Autodesk Inventor part; units mm, degrees
ref_plane "dia1_XY" through (0, 3.175, 0) normal (1, 0, 0) x (0, 0, -1)
ref_plane "dia1_YZ" through (0, 3.175, 0) normal (0, 0, -1) x (0, 1, 0)
ref_plane "dia1_ZX" through (0, 3.175, 0) normal (0, 1, 0) x (1, 0, 0)
sketch "Sketch_1" plane through (0, 0, 0) normal (0, 0, 1) x (1, 0, 0)
  line L0 (87.3252, 0) -> (0, 0)
  line L1 (0, 0) -> (0, 3.175)
  line L2 (0, 3.175) -> (65.8876, 3.175)
  line L3 (65.8876, 3.175) -> (65.8876, 9.6202)
  line L4 (65.8876, 9.6202) -> (87.3252, 9.6202)
  line L5 (87.3252, 9.6202) -> (87.3252, 0)
  line L6 (87.3252, 0) -> (0, 0)
revolve "Revolution1" add sketch "Sketch_1" angle 360 about axis through (87.3252, 0, 0) along (1, 0, 0)
sketch "Sketch_3" plane through (0, 0, 0) normal (0, 0, 1) x (1, 0, 0)
  line L0 (0, 0) -> (-12.7, 0)
  line L1 (-12.7, 0) -> (-12.7, 2.634)
  line L2 (-12.7, 2.634) -> (-12.159, 3.175)
  line L3 (-12.159, 3.175) -> (0, 3.175)
  line L4 (0, 3.175) -> (0, 0)
  line L5 (0, 0) -> (-12.7, 0)
revolve "Revolution2" add sketch "Sketch_3" angle 360 about axis through (0, 0, 0) along (1, 0, 0)
sketch "Sketch_30" plane through (0, 0, 0) normal (0, 0, 1) x (1, 0, 0)
  line L0 (0, 0) -> (-0.254, 0)
  line L1 (-0.254, 2.921) -> (0, 2.921)
  line L2 (0, 2.921) -> (0, 3.429)
  line L3 (0, 3.429) -> (-0.254, 3.429)
  line L4 (-0.254, 3.429) -> (-0.254, 2.921)
revolve "Revolution3" cut sketch "Sketch_30" angle 360 about axis through (0, 0, 0) along (1, 0, 0)
ref_plane "dia1_XY" through (0, 3.175, 0) normal (1, 0, 0) x (0, 0, -1)
ref_plane "dia1_YZ" through (0, 3.175, 0) normal (0, 0, -1) x (0, 1, 0)
ref_plane "dia1_ZX" through (0, 3.175, 0) normal (0, 1, 0) x (1, 0, 0)
ref_plane "dia12_XY" through (0, 0, 10.9537) normal (1, 0, 0) x (0, 0, -1)
ref_plane "dia12_YZ" through (0, 0, 10.9537) normal (0, 0, -1) x (0, 1, 0)
ref_plane "dia12_ZX" through (0, 0, 10.9537) normal (0, 1, 0) x (1, 0, 0)
ref_plane "dia2_XY" through (0, -3.175, 0) normal (1, 0, 0) x (0, 0, -1)
ref_plane "dia2_YZ" through (0, -3.175, 0) normal (0, 0, -1) x (0, 1, 0)
ref_plane "dia2_ZX" through (0, -3.175, 0) normal (0, 1, 0) x (1, 0, 0)
ref_plane "dia22_XY" through (0, 0, -10.9537) normal (1, 0, 0) x (0, 0, -1)
ref_plane "dia22_YZ" through (0, 0, -10.9537) normal (0, 0, -1) x (0, 1, 0)
ref_plane "dia22_ZX" through (0, 0, -10.9537) normal (0, 1, 0) x (1, 0, 0)
ref_plane "rl1_XY" through (-12.7, 0, 0) normal (1, 0, 0) x (0, 0, -1)
ref_plane "rl1_YZ" through (-12.7, 0, 0) normal (0, 0, -1) x (0, 1, 0)
ref_plane "rl1_ZX" through (-12.7, 0, 0) normal (0, 1, 0) x (1, 0, 0)
ref_plane "rl2_XY" through (0, 0, 0) normal (1, 0, 0) x (0, 0, -1)
ref_plane "rl2_YZ" through (0, 0, 0) normal (0, 0, -1) x (0, 1, 0)
ref_plane "rl2_ZX" through (0, 0, 0) normal (0, 1, 0) x (1, 0, 0)
ref_plane "rod_cp_XY" through (0, 0, 0) normal (1, 0, 0) x (0, 0, -1)
ref_plane "rod_cp_YZ" through (0, 0, 0) normal (0, 0, -1) x (0, 1, 0)
ref_plane "rod_cp_ZX" through (0, 0, 0) normal (0, 1, 0) x (1, 0, 0)
ref_plane "thd1_XY" through (-12.7, 3.175, 0) normal (1, 0, 0) x (0, 0, -1)
ref_plane "thd1_YZ" through (-12.7, 3.175, 0) normal (0, 0, -1) x (0, 1, 0)
ref_plane "thd1_ZX" through (-12.7, 3.175, 0) normal (0, 1, 0) x (1, 0, 0)
ref_plane "thd2_XY" through (-12.7, -3.175, 0) normal (1, 0, 0) x (0, 0, -1)
ref_plane "thd2_YZ" through (-12.7, -3.175, 0) normal (0, 0, -1) x (0, 1, 0)
ref_plane "thd2_ZX" through (-12.7, -3.175, 0) normal (0, 1, 0) x (1, 0, 0)
ref_plane "to_rod_clevis_XY" through (-16.764, 0, 0) normal (1, 0, 0) x (0, 0, -1)
ref_plane "to_rod_clevis_YZ" through (-16.764, 0, 0) normal (0, 0, -1) x (0, 1, 0)
ref_plane "to_rod_clevis_ZX" through (-16.764, 0, 0) normal (0, 1, 0) x (1, 0, 0)
properties part number "C-041-DP0000_rod"
Here's how the part is built. I have some questions about the finished solid (model axes, mm). A direction names the side the tool comes from. Round coordinates to 2 decimals unless told otherwise and drop trailing zeros. Order: outer loops, then holes, each group sorted by start corner. A loop starts at its lowest first (then second) coordinate and runs counter-clockwise, first axis right, second up. Notation, with made-up numbers: M 70.5,41.5 L 87.5,41.5 A29 cw 87.5,63.5 Z; hole C 19,-16 d4. An arc over 180 degrees is marked long. Return JSON: item names as keys, results as strings. Group by question number.
1. If we section it at C-C on x = 80: List the corners of the cut face in (y, z) for me.
2. If we section it at D-D on x = 59.5: List the corners of the cut face in (y, z) for me (3 decimals).
3. On a 3-axis mill with a long thin cutter (end or side, diameter ignored), from which of +Z, -Z, +X, -X, +Y, -Y can I reach the whole of each face in a straight line? I mean faces 1 (the face through (-12.7, 0, 0)), 2 (the face through (33.41, -0.69, -3.1)). Say none if no direction works.
4. If we section it at A-A on z = 0: List the corners of the cut face in (x, y) for me (3 decimals), then the cut area to 3 significant figures.
5. I'm going to push flat-ended pins straight in: pin 1 Ø1 at (x, y) = (46, -1) entering from +Z; pin 2 Ø3 at (x, z) = (1.5, -0.5) entering from -Y (3 decimals); pin 3 Ø8 at (x, z) = (41, -6.5) entering from -Y; pin 4 Ø2 at (x, z) = (19, 5.5) entering from +Y. Where does each tip first touch, or does it pass through?
6. Please list where these lines run through material, in increasing order: probe 1 along X at (y, z) = (-8, 3); probe 2 along Y at (x, z) = (20, -1.25); probe 3 along Y at (x, z) = (65, 0.25).
Reply:
{
 "1": {"outline": "C 0,0 d19.24"},
 "2": {"outline": "C 0,0 d6.35"},
 "3": {"face 1": "+Z, -Z, -X, +Y, -Y", "face 2": "-X"},
 "4": {"outline": "M -12.7,-2.634 L -12.159,-3.175 L -0.254,-3.175 L -0.254,-2.921 L 0,-2.921 L 0,-3.175 L 65.888,-3.175 L 65.888,-9.62 L 87.325,-9.62 L 87.325,9.62 L 65.888,9.62 L 65.888,3.175 L 0,3.175 L 0,2.921 L -0.254,2.921 L -0.254,3.175 L -12.159,3.175 L -12.7,2.634 Z", "area": "911 mm^2"},
 "5": {"pin 1": "z = 3.14", "pin 2": "y = -3.175", "pin 3": "y = -1.96", "pin 4": "through"},
 "6": {"probe 1": "65.89 to 87.33", "probe 2": "-2.92 to 2.92", "probe 3": "-3.17 to 3.17"}
}
